For this review, take the finished solid that the model builds, in its own axes (mm). A direction names the side the tool comes from. Coordinates: 2 decimals unless noted, no trailing zeros. Loops run counter-clockwise (first coordinate to the right, second up) from the corner with the lowest first, then second, coordinate; pieces in that order, holes last. Notation, with made-up numbers: M 88.25,-24 L 92.25,-24 A36 ccw 92.25,11 Z; hole C 51,-29 d6. An arc over 180 degrees is marked long. Answer as a JSON object with one key per item and string values. Group by question number.
Item 1: Add section B-B (z = -55). State the section outline as (x, y) points.
Item 2: Wall thickness on L1, parallel to X at y = 16.5, z = -36; L2, parallel to Z at x = 22.5, y = 13; L3, parallel to Z at x = 10, y = 21.5: over which ranges is each line inside the solid? List them lowest first. Write a range as from..to.
Item 3: Add section C-C (x = 31). State the section outline as (y, z) points.
Item 4: Add section A-A (y = 14). State the section outline as (x, z) points, then the cut area to 3 significant figures.
Item 5: Mouldability with a two-part tool opening along X and no side actions: class faces 1 (the face through (12, 17, -102.954)), 2 (the face through (33.954, 17, -34)), 3 (the face through (11, 0, -47)), 4 (the face through (-10.954, 17, -58)) as +X half, -X half, draft (parallel to the pull), parting line (faces both ways), or undercut.
Item 6: Tool access review of faces 5 (the face through (-10.954, 17, -35)), 6 (the face through (11, 17, 10.954)), 7 (the face through (33.954, 17, -11)): name each direction out of +Z, -Z, +X, -X, +Y, -Y from which nothing blocks a thin tool from reaching the whole face with its end or side.
Item 7: Insertion check: pin 1 (8 mm diameter, centred on y = 20.5, z = -77.5, fed in from -X); pin 2 (5 mm diameter, centred on y = 16.5, z = -38, fed in from +X); pin 3 (8 mm diameter, centred on x = 12.5, y = 9.5, fed in from +Z). Each pin has a flat end and moves straight along its axis. Give the tip position at first contact, or say it passes through.
from build123d import *

# Parameters (mm, degrees)
BOSS_EXTRUDE1_DEPTH = 34
BOSS_EXTRUDE2_DEPTH = 34


with BuildPart() as part:
    # Sketch1 → Boss-Extrude1 (new body)
    with BuildSketch(Plane(origin=(0, 0, 0), x_dir=(1, 0, 0), z_dir=(0, 1, 0))):
        with BuildLine():
            ThreePointArc((0, 11.5), (-8.131727984, -8.131727984), (11.5, 0))
            ThreePointArc((11.5, 0), (31.131727984, -8.131727984), (23, 11.5))
            ThreePointArc((23, 11.5), (34.5, 23), (23, 34.5))
            ThreePointArc((23, 34.5), (34.5, 46), (23, 57.5))
            ThreePointArc((23, 57.5), (34.5, 69), (23, 80.5))
            ThreePointArc((23, 80.5), (31.131727984, 100.131727984), (11.5, 92))
            ThreePointArc((11.5, 92), (-8.131727984, 100.131727984), (0, 80.5))
            ThreePointArc((0, 80.5), (-11.5, 69), (0, 57.5))
            ThreePointArc((0, 57.5), (-11.5, 46), (0, 34.5))
            ThreePointArc((0, 34.5), (-11.5, 23), (0, 11.5))
        make_face()
    extrude(amount=BOSS_EXTRUDE1_DEPTH)

    # Sketch2 → Boss-Extrude2 (add)
    with BuildSketch(Plane(origin=(0, 34, 0), x_dir=(1, 0, 0), z_dir=(0, 1, 0))):
        Polygon((-10.95445115, 88.5), (-10.95445115, 72.5), (-10.95445115, 3.5), (3.5, -10.95445115), (19.5, -10.95445115), (33.95445115, -3.5), (33.95445115, 88.5), (19.5, 102.95445115), (3.5, 102.95445115), align=None)
    extrude(amount=-BOSS_EXTRUDE2_DEPTH)


solid = part.part
From the geometry:
{
 "1": {"outline": "M -10.95,0 L 33.95,0 L 33.95,34 L -10.95,34 Z"},
 "2": {"L1": "x = -10.95..33.95", "L2": "z = -103.49..11.49", "L3": "z = -102.95..10.95"},
 "3": {"outline": "M 0,-100.26 L 34,-100.26 L 34,8.26 L 0,8.26 Z"},
 "4": {"outline": "M -10.95,-88.5 A11.5 ccw 3.5,-102.95 L 19.5,-102.95 A11.5 ccw 33.95,-88.5 L 33.95,-72.5 A11.5 ccw 33.95,-65.5 L 33.95,-49.5 A11.5 ccw 33.95,-42.5 L 33.95,-26.5 A11.5 ccw 33.95,-19.5 L 33.95,-3.5 A11.5 ccw 19.5,10.95 L 3.5,10.95 A11.5 ccw -10.95,-3.5 L -10.95,-19.5 A11.5 ccw -10.95,-26.5 L -10.95,-42.5 A11.5 ccw -10.95,-49.5 L -10.95,-65.5 A11.5 ccw -10.95,-72.5 Z", "area": "5,080 mm²"},
 "5": {"face 1": "undercut", "face 2": "+X half", "face 3": "draft", "face 4": "-X half"},
 "6": {"face 5": "-X, +Y, -Y", "face 6": "+Z, +Y, -Y", "face 7": "+X, +Y, -Y"},
 "7": {"pin 1": "stops at x = -10.95", "pin 2": "stops at x = 33.95", "pin 3": "stops at z = 10.95"}
}
